Work out the finished part from the listing and answer in its coordinate system (mm). A direction names the side the tool comes from. Coordinates: 2 decimals unless noted, no trailing zeros. Write each loop counter-clockwise with the first axis right and the second up, starting at its lowest first coordinate (ties: lowest second). Pieces come first, ordered by that corner, then holes. Notation, with made-up numbers: (-39, -26) - (13, -26) arc R28 ccw to (13, -2) - close; hole circle Ø2 at (69, 62.25). An arc over 180 degrees is marked (long way). Use CSV: the item, a comma, the result in double quotes. Start each with the question number.
from build123d import *

# Parameters (mm, degrees)
CROQUIS1_R                                           = 132.5
SALIENTE_EXTRUIR1_DEPTH                              = 5
AVELLANADO_PARA_TORNILLO_CON_CABEZA_PLAN_D           = 6.6
AVELLANADO_PARA_TORNILLO_CON_CABEZA_PLAN_CSINK_D     = 12.6
AVELLANADO_PARA_TORNILLO_CON_CABEZA_PLAN_CSINK_ANGLE = 90
AVELLANADO_PARA_TORNILLO_CON_CABEZA_2_D              = 2.4
AVELLANADO_PARA_TORNILLO_CON_CABEZA_2_CSINK_D        = 4.4
AVELLANADO_PARA_TORNILLO_CON_CABEZA_2_CSINK_ANGLE    = 90
CORTAR_EXTRUIR1_DEPTH                                = 5
CROQUIS20_W                                          = 70
CROQUIS20_H                                          = 35
SALIENTE_EXTRUIR2_DEPTH                              = 51
CORTAR_EXTRUIR3_REACH                                = 274.422
TALADRO_DE_MARGEN_PARA_M131_D                        = 16
CORTAR_EXTRUIR4_REACH                                = 208.536
CROQUIS24_W                                          = 25
CROQUIS24_H                                          = 51
CHAFL_N1_SIZE                                        = 3
CROQUIS25_W                                          = 71.5
CROQUIS25_H                                          = 25
CORTAR_EXTRUIR5_DEPTH                                = 5
TALADRO_DE_MARGEN_PARA_M31_D                         = 3.6
CROQUIS26_W                                          = 6
CROQUIS26_H                                          = 19
CORTAR_EXTRUIR6_DEPTH                                = 3.5
CROQUIS27_W                                          = 50
CROQUIS27_H                                          = 8
CORTAR_EXTRUIR7_DEPTH                                = 2
CROQUIS28_W                                          = 13
CROQUIS28_H                                          = 20
CORTAR_EXTRUIR8_DEPTH                                = 5
CROQUIS29_R                                          = 6.5
CORTAR_EXTRUIR9_DEPTH                                = 5
AVELLANADO_PARA_TORNILLO_CON_CABEZA_3_D              = 3.6
AVELLANADO_PARA_TORNILLO_CON_CABEZA_3_CSINK_D        = 6.3
AVELLANADO_PARA_TORNILLO_CON_CABEZA_3_CSINK_ANGLE    = 90
AVELLANADO_PARA_TORNILLO_CON_CABEZA_4_D              = 3.6
AVELLANADO_PARA_TORNILLO_CON_CABEZA_4_CSINK_D        = 6.3
AVELLANADO_PARA_TORNILLO_CON_CABEZA_4_CSINK_ANGLE    = 90
AVELLANADO_PARA_TORNILLO_CON_CABEZA_5_D              = 3.6
AVELLANADO_PARA_TORNILLO_CON_CABEZA_5_CSINK_D        = 6.3
AVELLANADO_PARA_TORNILLO_CON_CABEZA_5_CSINK_ANGLE    = 90
AVELLANADO_PARA_TORNILLO_CON_CABEZA_6_D              = 3.6
AVELLANADO_PARA_TORNILLO_CON_CABEZA_6_CSINK_D        = 6.3
AVELLANADO_PARA_TORNILLO_CON_CABEZA_6_CSINK_ANGLE    = 90
AVELLANADO_PARA_TORNILLO_CON_CABEZA_7_D              = 3.6
AVELLANADO_PARA_TORNILLO_CON_CABEZA_7_CSINK_D        = 6.3
AVELLANADO_PARA_TORNILLO_CON_CABEZA_7_CSINK_ANGLE    = 90
CROQUIS41_R                                          = 3.75
SALIENTE_EXTRUIR3_DEPTH                              = 15
CROQUIS42_R                                          = 2
CORTAR_EXTRUIR10_DEPTH                               = 6.5


with BuildPart() as part:
    # Croquis1 → Saliente-Extruir1 (new body)
    with BuildSketch(Plane(origin=(0, 0, 0), x_dir=(1, 0, 0), z_dir=(0, 1, 0))):
        with Locations(Location((0, 0, 0), (0, 0, 270))):
            Circle(CROQUIS1_R)
    extrude(amount=SALIENTE_EXTRUIR1_DEPTH)

    # Avellanado para tornillo con cabeza plan (through all)
    with Locations(Plane(origin=(0, 5, 0), x_dir=(1, 0, 0), z_dir=(0, 1, 0))):
        with Locations((-87, -45), (87, -45), (87, 45), (-87, 45)):
            CounterSinkHole(AVELLANADO_PARA_TORNILLO_CON_CABEZA_PLAN_D / 2, AVELLANADO_PARA_TORNILLO_CON_CABEZA_PLAN_CSINK_D / 2, counter_sink_angle=AVELLANADO_PARA_TORNILLO_CON_CABEZA_PLAN_CSINK_ANGLE)

    # Avellanado para tornillo con cabeza  2 (through all)
    with Locations(Plane(origin=(0, 0, 0), x_dir=(-1, 0, 0), z_dir=(0, -1, 0))):
        with Locations((-28.5, 25), (28.5, 31), (-28.5, -25), (28.5, -31)):
            CounterSinkHole(AVELLANADO_PARA_TORNILLO_CON_CABEZA_2_D / 2, AVELLANADO_PARA_TORNILLO_CON_CABEZA_2_CSINK_D / 2, counter_sink_angle=AVELLANADO_PARA_TORNILLO_CON_CABEZA_2_CSINK_ANGLE)

    # Croquis18 → Cortar-Extruir1 (cut)
    with BuildSketch(Plane.XZ):
        with BuildLine():
            Line((-15, 0), (15, 0))
            ThreePointArc((15, 0), (0, -15), (-15, 0))
        make_face()
    extrude(amount=-CORTAR_EXTRUIR1_DEPTH, mode=Mode.SUBTRACT)

    # Croquis20 → Saliente-Extruir2 (add)
    with BuildSketch(Plane.XZ):
        with Locations((65, 0)):
            Rectangle(CROQUIS20_W, CROQUIS20_H)
        with Locations((-65, 0)):
            Rectangle(CROQUIS20_W, CROQUIS20_H)
    extrude(amount=SALIENTE_EXTRUIR2_DEPTH)

    # Cortar-Extruir3: up to this face of the body (flat: up to its plane)
    cortar_extruir3_end = Plane(part.part.faces().sort_by_distance((-100, -25.5, 0))[0])
    # Croquis21 → Cortar-Extruir3 (cut, up to the picked face)
    with BuildSketch(Plane(origin=(100, 0, 0), x_dir=(0, 0, -1), z_dir=(1, 0, 0)), mode=Mode.PRIVATE) as cortar_extruir3_sk1:
        with BuildLine():
            Line((-14.1, -51), (14.1, -51))
            ThreePointArc((14.1, -51), (0, -36.9), (-14.1, -51))
        make_face()
    cortar_extruir3_tool1 = split(extrude(cortar_extruir3_sk1.sketch, amount=-CORTAR_EXTRUIR3_REACH, mode=Mode.PRIVATE), bisect_by=cortar_extruir3_end, keep=Keep.BOTH, mode=Mode.PRIVATE)
    # Croquis21 → Cortar-Extruir3 (cut, up to the picked face)
    with BuildSketch(Plane(origin=(100, 0, 0), x_dir=(0, 0, -1), z_dir=(1, 0, 0)), mode=Mode.PRIVATE) as cortar_extruir3_sk2:
        Polygon((-3, -6), (-13, -6), (-13, -36), (-3, -24.082464074), align=None)
    cortar_extruir3_tool2 = split(extrude(cortar_extruir3_sk2.sketch, amount=-CORTAR_EXTRUIR3_REACH, mode=Mode.PRIVATE), bisect_by=cortar_extruir3_end, keep=Keep.BOTH, mode=Mode.PRIVATE)
    # Croquis21 → Cortar-Extruir3 (cut, up to the picked face)
    with BuildSketch(Plane(origin=(100, 0, 0), x_dir=(0, 0, -1), z_dir=(1, 0, 0)), mode=Mode.PRIVATE) as cortar_extruir3_sk3:
        Polygon((3, -6), (3, -24.082464074), (13, -36), (13, -6), align=None)
    cortar_extruir3_tool3 = split(extrude(cortar_extruir3_sk3.sketch, amount=-CORTAR_EXTRUIR3_REACH, mode=Mode.PRIVATE), bisect_by=cortar_extruir3_end, keep=Keep.BOTH, mode=Mode.PRIVATE)
    add(cortar_extruir3_tool1.solids().sort_by(Axis((100, -45.015774, 0), (-1, 0, 0)))[0], mode=Mode.SUBTRACT)
    add(cortar_extruir3_tool2.solids().sort_by(Axis((100, -18.266769, 8.413094), (-1, 0, 0)))[0], mode=Mode.SUBTRACT)
    add(cortar_extruir3_tool3.solids().sort_by(Axis((100, -18.266769, -8.413094), (-1, 0, 0)))[0], mode=Mode.SUBTRACT)

    # Taladro de margen para M131 (through all)
    with Locations(Plane(origin=(0, 5, 0), x_dir=(1, 0, 0), z_dir=(0, 1, 0))):
        with Locations((75, -60)):
            Hole(TALADRO_DE_MARGEN_PARA_M131_D / 2)

    # Cortar-Extruir4: up to this face of the body (flat: up to its plane)
    cortar_extruir4_end = Plane(part.part.faces().sort_by_distance((-65, -25.5, -17.5))[0])
    # Croquis24 → Cortar-Extruir4 (cut, up to the picked face)
    with BuildSketch(Plane.XY.offset(17.5), mode=Mode.PRIVATE) as cortar_extruir4_sk1:
        with Locations((-65, -25.5)):
            Rectangle(CROQUIS24_W, CROQUIS24_H)
    cortar_extruir4_tool1 = split(extrude(cortar_extruir4_sk1.sketch, amount=-CORTAR_EXTRUIR4_REACH, mode=Mode.PRIVATE), bisect_by=cortar_extruir4_end, keep=Keep.BOTH, mode=Mode.PRIVATE)
    # Croquis24 → Cortar-Extruir4 (cut, up to the picked face)
    with BuildSketch(Plane.XY.offset(17.5), mode=Mode.PRIVATE) as cortar_extruir4_sk2:
        with Locations((65, -25.5)):
            Rectangle(CROQUIS24_W, CROQUIS24_H)
    cortar_extruir4_tool2 = split(extrude(cortar_extruir4_sk2.sketch, amount=-CORTAR_EXTRUIR4_REACH, mode=Mode.PRIVATE), bisect_by=cortar_extruir4_end, keep=Keep.BOTH, mode=Mode.PRIVATE)
    add(cortar_extruir4_tool1.solids().sort_by(Axis((-65, -25.5, 17.5), (0, 0, -1)))[0], mode=Mode.SUBTRACT)
    add(cortar_extruir4_tool2.solids().sort_by(Axis((65, -25.5, 17.5), (0, 0, -1)))[0], mode=Mode.SUBTRACT)

    # Chaflán1
    chafl_n1_edges = [part.edges().sort_by_distance(p)[0] for p in [
        (-41.25, 0, -17.5),
        (-88.75, 0, 17.5),
        (88.75, 0, -17.5),
        (41.25, 0, 17.5),
        (100, 0, 0),
        (88.75, 0, 17.5),
        (30, 0, 0),
        (41.25, 0, -17.5),
        (-30, 0, 0),
        (-41.25, 0, 17.5),
        (-100, 0, 0),
        (-88.75, 0, -17.5),
    ]]
    chamfer(chafl_n1_edges, length=CHAFL_N1_SIZE)

    # Croquis25 → Cortar-Extruir5 (cut)
    with BuildSketch(Plane(origin=(0, 5, 0), x_dir=(1, 0, 0), z_dir=(0, 1, 0))):
        with Locations((0, -89.5)):
            Rectangle(CROQUIS25_W, CROQUIS25_H)
    extrude(amount=-CORTAR_EXTRUIR5_DEPTH, mode=Mode.SUBTRACT)

    # Taladro de margen para M31 (through all)
    with Locations(Plane(origin=(0, 0, 0), x_dir=(-1, 0, 0), z_dir=(0, -1, 0))):
        with Locations((37.25, -104), (-37.25, -104), (37.25, -73.5), (-37.25, -73.5)):
            Hole(TALADRO_DE_MARGEN_PARA_M31_D / 2)

    # Croquis26 → Cortar-Extruir6 (cut)
    with BuildSketch(Plane.XZ):
        with Locations((38.75, 89.5)):
            Rectangle(CROQUIS26_W, CROQUIS26_H)
    extrude(amount=-CORTAR_EXTRUIR6_DEPTH, mode=Mode.SUBTRACT)

    # Croquis27 → Cortar-Extruir7 (cut)
    with BuildSketch(Plane.XZ):
        with Locations((-8.25, 73)):
            Rectangle(CROQUIS27_W, CROQUIS27_H)
    extrude(amount=-CORTAR_EXTRUIR7_DEPTH, mode=Mode.SUBTRACT)

    # Croquis28 → Cortar-Extruir8 (cut)
    with BuildSketch(Plane.XZ):
        with Locations((-55, 87.5)):
            Rectangle(CROQUIS28_W, CROQUIS28_H)
    extrude(amount=-CORTAR_EXTRUIR8_DEPTH, mode=Mode.SUBTRACT)

    # Croquis29 → Cortar-Extruir9 (cut)
    with BuildSketch(Plane(origin=(0, 5, 0), x_dir=(1, 0, 0), z_dir=(0, 1, 0))):
        with Locations(Location((-75, -60, 0), (0, 0, 270))):
            Circle(CROQUIS29_R)
    extrude(amount=-CORTAR_EXTRUIR9_DEPTH, mode=Mode.SUBTRACT)

    # Avellanado para tornillo con cabeza  3 (through all)
    with Locations(Plane(origin=(0, 0, 0), x_dir=(-1, 0, 0), z_dir=(0, -1, 0))):
        with Locations((65, 40.5), (65, -40.5), (-65, -40.5), (-65, 40.5)):
            CounterSinkHole(AVELLANADO_PARA_TORNILLO_CON_CABEZA_3_D / 2, AVELLANADO_PARA_TORNILLO_CON_CABEZA_3_CSINK_D / 2, counter_sink_angle=AVELLANADO_PARA_TORNILLO_CON_CABEZA_3_CSINK_ANGLE)

    # Avellanado para tornillo con cabeza  4 (through all)
    with Locations(Plane(origin=(0, 0, 0), x_dir=(-1, 0, 0), z_dir=(0, -1, 0))):
        with Locations((56.74, 97.5), (20, 60.12)):
            CounterSinkHole(AVELLANADO_PARA_TORNILLO_CON_CABEZA_4_D / 2, AVELLANADO_PARA_TORNILLO_CON_CABEZA_4_CSINK_D / 2, counter_sink_angle=AVELLANADO_PARA_TORNILLO_CON_CABEZA_4_CSINK_ANGLE)

    # Avellanado para tornillo con cabeza  5 (through all)
    with Locations(Plane(origin=(0, 0, 0), x_dir=(-1, 0, 0), z_dir=(0, -1, 0))):
        with Locations((-28, 73.18), (-45, 40)):
            CounterSinkHole(AVELLANADO_PARA_TORNILLO_CON_CABEZA_5_D / 2, AVELLANADO_PARA_TORNILLO_CON_CABEZA_5_CSINK_D / 2, counter_sink_angle=AVELLANADO_PARA_TORNILLO_CON_CABEZA_5_CSINK_ANGLE)

    # Avellanado para tornillo con cabeza  6 (through all)
    with Locations(Plane(origin=(0, 0, 0), x_dir=(-1, 0, 0), z_dir=(0, -1, 0))):
        with Locations((16.59, -57), (-16.59, -40)):
            CounterSinkHole(AVELLANADO_PARA_TORNILLO_CON_CABEZA_6_D / 2, AVELLANADO_PARA_TORNILLO_CON_CABEZA_6_CSINK_D / 2, counter_sink_angle=AVELLANADO_PARA_TORNILLO_CON_CABEZA_6_CSINK_ANGLE)

    # Avellanado para tornillo con cabeza  7 (through all)
    with Locations(Plane(origin=(0, 0, 0), x_dir=(-1, 0, 0), z_dir=(0, -1, 0))):
        with Locations((11.5, 22.5), (-11.5, 35.5)):
            CounterSinkHole(AVELLANADO_PARA_TORNILLO_CON_CABEZA_7_D / 2, AVELLANADO_PARA_TORNILLO_CON_CABEZA_7_CSINK_D / 2, counter_sink_angle=AVELLANADO_PARA_TORNILLO_CON_CABEZA_7_CSINK_ANGLE)

    # Croquis41 → Saliente-Extruir3 (add)
    with BuildSketch(Plane(origin=(0, 0, 0), x_dir=(-1, 0, 0), z_dir=(0, -1, 0))):
        with Locations(Location((7.753, -5.24, 0), (0, 0, 270))):
            Circle(CROQUIS41_R)
        with Locations(Location((-7.807, -5.24, 0), (0, 0, 270))):
            Circle(CROQUIS41_R)
    extrude(amount=SALIENTE_EXTRUIR3_DEPTH)

    # Croquis42 → Cortar-Extruir10 (cut)
    with BuildSketch(Plane(origin=(0, -15, 0), x_dir=(-1, 0, 0), z_dir=(0, -1, 0))):
        with Locations(Location((7.753, -5.24, 0), (0, 0, 90))):
            Circle(CROQUIS42_R)
        with Locations(Location((-7.807, -5.24, 0), (0, 0, 90))):
            Circle(CROQUIS42_R)
    extrude(amount=-CORTAR_EXTRUIR10_DEPTH, mode=Mode.SUBTRACT)


solid = part.part
Item 1: A cutting plane is placed at B-B (z = 84). Determine the outline of the cut face in (x, y).
Item 2: Determine the mould class of faces 5 (the face through (2, 0, -31)), 6 (the face through (39.8, 2.46, 126.38)), 7 (the face through (41.41, -29.96, -7.93)), 8 (the face through (41, -27, -17.5)) for opening direction Z: +Z half, -Z half, draft (parallel to the pull), parting line (faces both ways), or undercut.
Item 3: Each of these flat-tipped pins is pushed along its axis until it touches: pin 1 (1 mm diameter, centred on y = -32, z = 4, fed in from -X); pin 2 (14.5 mm diameter, centred on x = 85.5, y = -13, fed in from +Z); pin 3 (2.5 mm diameter, centred on x = -1.5, z = 74, fed in from -Y). Where does it stop, or does it pass through?
Item 4: Which of the six approach directions +Z, -Z, +X, -X, +Y, -Y give full straight-line access (tool end or side, diameter ignored) to faces 1 (the face through (-89, -21, 13)), 2 (the face through (-41, -6, 8)), 3 (the face through (100, -27, 0)), 4 (the face through (77.5, -20, 0))?
Item 5: Straight lines are drawn through the part: probe 1 along Z at (x, y) = (87, -22); probe 2 along X at (y, z) = (2, -97); probe 3 along Z at (x, y) = (-28.5, 3.2). For each, find the intervals that lie inside material, in ascending order. Write a range as [from, to].
Item 6: A cutting plane is placed at C-C (z = -84.5). Determine the outline of the cut face in (x, y).
Item 7: A cutting plane is placed at A-A (y = -19.5). Count the separate pieces of the cut face and the enclosed holes in it, then the cut area to 3 significant figures.
Calculated:
1,outline,"(-102.47, 0) - (-61.5, 0) - (-61.5, 5) - (-102.47, 5) - close; (-48.5, 0) - (-35.75, 0) - (-35.75, 5) - (-48.5, 5) - close; (35.75, 3.5) - (41.75, 3.5) - (41.75, 0) - (102.47, 0) - (102.47, 5) - (35.75, 5) - close"
2,face 5,"draft"
2,face 6,"parting line"
2,face 7,"undercut"
2,face 8,"-Z half"
3,pin 1,"stops at x = -100"
3,pin 2,"stops at z = 17.5"
3,pin 3,"stops at y = 2"
4,face 1,"+X, -X"
4,face 2,"-X"
4,face 3,"+Z, -Z, +X, -Y"
4,face 4,"+Z, -Z, -Y"
5,probe 1,"z = [-17.5, -13], [-3, 3], [13, 17.5]"
5,probe 2,"x = [-90.26, -58.47], [-55.01, 90.26]"
5,probe 3,"z = [-129.4, -32.2], [-29.8, 29.8], [32.2, 77], [102, 129.4]"
6,outline,"(-102.06, 0) - (102.06, 0) - (102.06, 5) - (-102.06, 5) - close"
7,separate pieces,"12"
7,enclosed holes,"0"
7,area,"1,350 mm²"
